Part model, mm, in its own coordinate system. Face numbers are marked on the shaded views. A direction names the side the tool comes from. Give positions to 0.01 mm unless a question says otherwise; leave off trailing zeros. Write each loop counter-clockwise with the first axis right and the second up, starting at its lowest first coordinate (ties: lowest second). Pieces come first, ordered by that corner, then holes.
from build123d import *

# Parameters (mm, degrees)
SKETCH1_R           = 0.675
BOSS_EXTRUDE1_DEPTH = 2


with BuildPart() as part:
    # Sketch1 → Boss-Extrude1 (new body)
    with BuildSketch(Plane(origin=(0, 0, 0), x_dir=(1, 0, 0), z_dir=(0, 1, 0))):
        with BuildLine():
            Line((-1.772653955, -0.31256672), (0, 0))
            Line((0, 0), (0, 1.45))
            Line((0, 1.45), (-0.845723359, 1.142181871))
            Line((-0.845723359, 1.142181871), (-0.845723359, 4.742181871))
            Line((-0.845723359, 4.742181871), (0, 4.434363742))
            Line((0, 4.434363742), (0, 6.35))
            Line((0, 6.35), (-2.855942484, 6.853579715))
            add(Edge.make_bspline(
                [(-4.214404462, 6.242429297), (-3.782908861, 7.104554386), (-2.855942484, 6.853579715)],
                knots=[0, 0, 0, 1, 1, 1], degree=2))
            add(Edge.make_bspline(
                [(-2.646853101, 0.302878761), (-4.217046525, 3.042629381), (-4.214404462, 6.242429297)],
                knots=[0, 0, 0, 1, 1, 1], degree=2))
            add(Edge.make_bspline(
                [(-1.772653955, -0.31256672), (-2.342932983, -0.342253748), (-2.646853101, 0.302878761)],
                knots=[0, 0, 0, 1, 1, 1], degree=2))
        make_face()
        with Locations((-1.845723359, 2.942181871)):
            Circle(SKETCH1_R, mode=Mode.SUBTRACT)
    extrude(amount=BOSS_EXTRUDE1_DEPTH)


solid = part.part
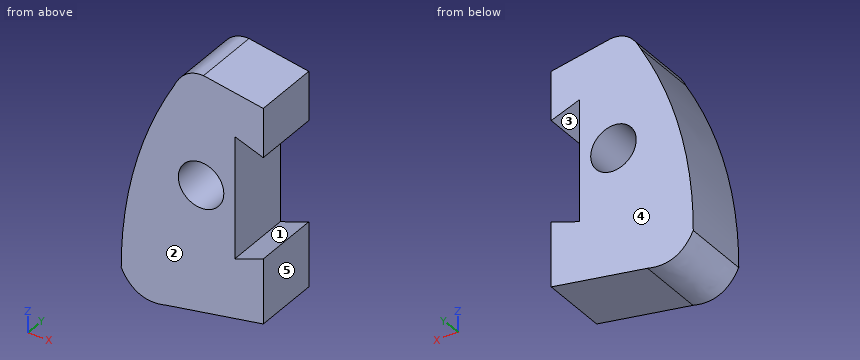
1) Saw through at A-A (x = -0.25). Write the cut outline in (y, z).
Check result:
outline: (0, -6.39) - (2, -6.39) - (2, -4.53) - (0, -4.53) - close; (0, -1.36) - (2, -1.36) - (2, 0.04) - (0, 0.04) - close
2) Mould opens along X. For the marked faces 3, 4 and 5 say: +X half, -X half, draft (parallel to the pull), parting line (faces both ways), or undercut.
Check result:
face 3: undercut
face 4: draft
face 5: +X half
3) Drill centre lines: L1, parallel to X at y = 1.95, z = -3.5; L2, parallel to X at y = 0.9, z = -3; L3, parallel to Z at x = -0.5, y = 1.35. Where is each one in solid material? Low to high.
Check result:
L1: x = -3.91 to -2.23, -1.47 to -0.85
L2: x = -3.78 to -2.52, -1.17 to -0.85
L3: z = -6.44 to -4.62, -1.27 to 0.09
4) Flat gauge pins, fed straight in: P1, Ø1, axis at y = 1, z = -2.5, coming from the +X side; P2, Ø1, axis at x = -0.5, y = 0.5, coming from the +Z side; P3, Ø1, axis at y = 0.5, z = -2, coming from the -X side. Where does each tip first touch, or does it go through?
Check result:
P1: stops at x = -0.85
P2: stops at z = 0.18
P3: stops at x = -3.63
5) 3-axis set-ups, long thin cutter, end or side, ignore diameter. For the marked faces 1 and 2: which of +Z, -Z, +X, -X, +Y, -Y reach the whole face in a straight line?
Check result:
face 1: +Y, -Y
face 2: +Z, -Z, +X, -X, -Y
